Design review of the part shown in the three views and the two pictorial views. Dimensions are in mm from the part's minimum x, y and z. A direction names the side the tool comes from. Round coordinates to 2 decimals unless told otherwise and drop trailing zeros. Loops run counter-clockwise (first coordinate to the right, second up) from the corner with the lowest first, then second, coordinate; pieces in that order, holes last. Notation, with made-up numbers: (-31.5, 54) - (-27.5, 54) arc R22 ccw to (-27.5, 65) - close; hole circle Ø5 at (86, 62). An arc over 180 degrees is marked (long way). Return JSON: item names as keys, results as strings. Group by question number.
(1) For the marked faces 1 and 2, list the 3-axis set-ups (+Z, -Z, +X, -X, +Y, -Y) from which the entire face can be reached by the end or side of a thin tool; tool diameter is ignored.
(2) We need section B-B, the plane z = 24. Write out the cut boundary in (x, y).
(3) We need section C-C, the plane y = 35. Write out the cut boundary in (x, z).
(4) We need section A-A, the plane x = 34. Write out the cut boundary in (y, z).
(5) Wall thickness on L1, parallel to Y at x = 17, z = 15; L2, parallel to Z at x = 4, y = 29; L3, parallel to X at y = 33, z = 23: over which ranges is each line inside the solid? List them lowest first. Write a range as [from, to].
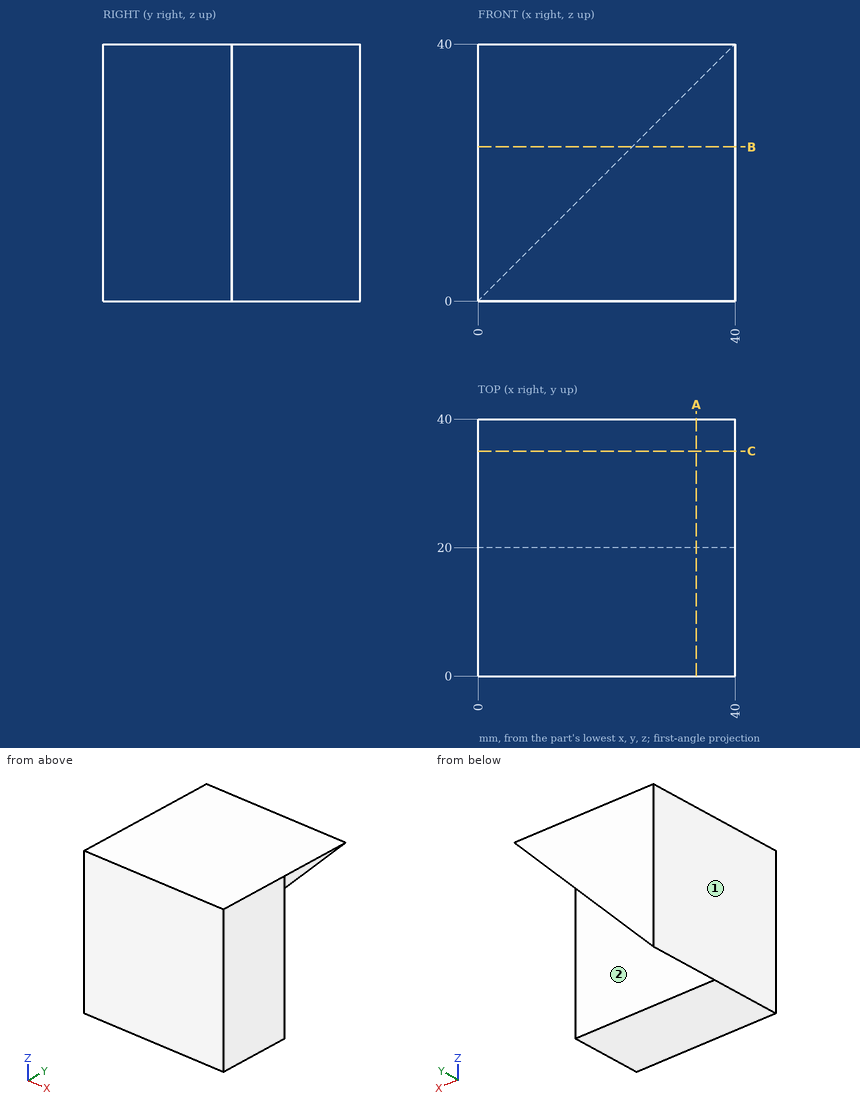
Solutions:
{
 "1": {"face 1": "+Z, -Z, -X, +Y, -Y", "face 2": "-Z, +X, +Y"},
 "2": {"outline": "(0, 0) - (40, 0) - (40, 20) - (24, 20) - (24, 40) - (0, 40) - close"},
 "3": {"outline": "(0, 0) - (40, 40) - (0, 40) - close"},
 "4": {"outline": "(0, 0) - (20, 0) - (20, 34) - (40, 34) - (40, 40) - (0, 40) - close"},
 "5": {"L1": "[0, 20]", "L2": "[4, 40]", "L3": "[0, 23]"}
}
